```python
from build123d import *


with BuildPart() as part:
    # Çizim1 → Döndür1 (revolve)
    with BuildSketch(Plane.XY, mode=Mode.PRIVATE) as d_nd_r1_sk:
        with BuildLine():
            Line((0, 6.55), (0, 6.05))
            Line((0, 6.05), (0.378679656, 6.05))
            ThreePointArc((0.378679656, 6.05), (0.952704805, 5.935819299), (1.439339828, 5.610660172))
            Line((1.439339828, 5.610660172), (2.097487373, 4.952512627))
            ThreePointArc((2.097487373, 4.952512627), (2.211035546, 4.876642164), (2.344974747, 4.85))
            Line((2.344974747, 4.85), (2.55, 4.85))
            Line((2.55, 4.85), (2.55, 6.55))
            Line((2.55, 6.55), (0, 6.55))
        make_face()
    revolve(d_nd_r1_sk.sketch.rotate(Axis((0, 0, 0), (1, 0, 0)), 90), axis=Axis((0, 0, 0), (1, 0, 0)))

    # Pah1: read off the stored shape, not the designer's step
    # Pah1 outline → Pah1 (revolve, cut)
    with BuildSketch(Plane.YX):
        Polygon((4.887395483, 2.187563133), (5.110684424, 2.55), (4.85, 2.55), (4.85, 2.187563133), align=None)
        Polygon((6.55, 2.55), (6.3, 2.55), (6.55, 2.3), align=None)
        Polygon((6.55, 0), (6.55, 0.25), (6.3, 0), align=None)
    revolve(axis=Axis((0, 0, 0), (1, 0, 0)), mode=Mode.SUBTRACT)


solid = part.part
```
Source: CAD feature listing. Evaluate the final solid. Frame: model axes, mm. Round coordinates to 2 decimals unless told otherwise and drop trailing zeros. Loops run counter-clockwise (first coordinate to the right, second up) from the corner with the lowest first, then second, coordinate; pieces in that order, holes last.
1. Section query A-A on y = 0. Output: boundary loops of the cut face in (x, z), and give its area (3 significant figures).
2. Section query D-D on x = 1. Output: boundary loops of the cut face in (y, z), and give its area (3 significant figures).
3. Ray query, L1, parallel to Y at x = 1.5, z = 2.5; L2, parallel to Z at x = 0.5, y = -0.25; L3, parallel to Z at x = 0.7, y = -4.5. Return the intervals inside material, ascending.
4. Mould query, pull axis Y, two halves, no side actions, for faces 1 (the flat face through (2.55, -5.2, 1)), 2 (the cylindrical face through (0.19, -1.82, 5.77)), 3 (the cylindrical face through (1.261, -1.967, 6.248)). Classes: released by +Y, released by -Y, zero draft, split by the parting line, or undercut.
5. Section query C-C on x = 1.85. Output: boundary loops of the cut face in (y, z), and give its area (3 significant figures).
Answers below:
1. outline: (0, -6.3) - (0.25, -6.55) - (2.3, -6.55) - (2.55, -6.3) - (2.55, -5.11) - (2.19, -4.89) arc R0.35 ccw to (2.1, -4.95) - (1.44, -5.61) arc R1.5 cw to (0.38, -6.05) - (0, -6.05) - close; (0, 6.05) - (0.38, 6.05) arc R1.5 cw to (1.44, 5.61) - (2.1, 4.95) arc R0.35 ccw to (2.19, 4.89) - (2.55, 5.11) - (2.55, 6.3) - (2.3, 6.55) - (0.25, 6.55) - (0, 6.3) - close
1. area: 4.69 mm2
2. outline: circle Ø13.1 at (0, 0); hole circle Ø11.83 at (0, 0)
2. area: 24.9 mm2
3. L1: y = -6.05 to -4.96, 4.96 to 6.05
3. L2: z = -6.55 to -6.04, 6.04 to 6.55
3. L3: z = -4.76 to -3.99, 3.99 to 4.76
4. face 1: zero draft
4. face 2: undercut
4. face 3: split by the parting line
5. outline: circle Ø13.1 at (0, 0); hole circle Ø10.4 at (0, 0)
5. area: 49.8 mm2
